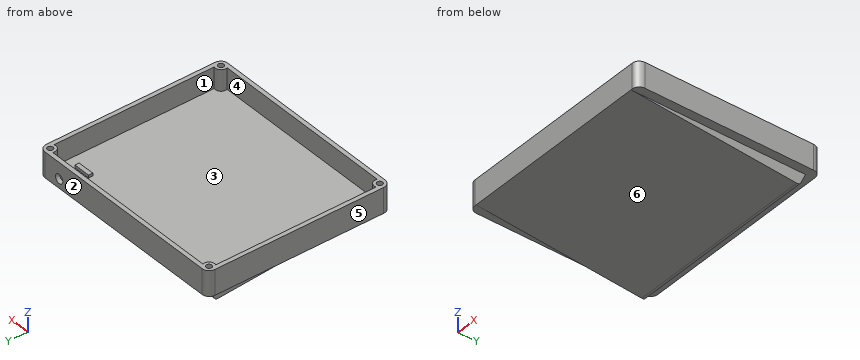
from build123d import *

# Parameters (mm, degrees)
LEFT_BODY_PAD_DEPTH            = 18
LEFT_BODY_CAVITY_POCKET_DEPTH  = 15
LEFT_BODY_BOSSES_R             = 4
LEFT_BODY_BOSS_PAD_DEPTH       = 15
LEFT_BODY_INSERT_HOLES_R       = 2
LEFT_BODY_INSERT_POCKETS_DEPTH = 7
LEFT_BODY_REST_PAD_DEPTH       = 68.531175
LEFT_BODY_REST_FILLET_R        = 3
LEFT_JACK_HOLE_R               = 3.25
LEFT_JACK_HOLE_POCKET_DEPTH    = 3.2
LEFT_JACK_STOP_W               = 12
LEFT_JACK_STOP_H               = 3
LEFT_JACK_STOP_PAD_DEPTH       = 2


with BuildPart() as part:
    # Left_Body_Outline → Left_Body_Pad (new body)
    with BuildSketch(Plane.XY.offset(-18)):
        with BuildLine():
            Line((-0.38035, -5.791), (138.682, -5.791))
            ThreePointArc((138.682, -5.791), (142.217534, -4.326534), (143.682, -0.791))
            Line((143.682, -0.791), (143.682, 119.971))
            ThreePointArc((143.682, 119.971), (142.217534, 123.506534), (138.682, 124.971))
            Line((138.682, 124.971), (-0.38035, 124.971))
            ThreePointArc((-0.38035, 124.971), (-3.915884, 123.506534), (-5.38035, 119.971))
            Line((-5.38035, 119.971), (-5.38035, -0.791))
            ThreePointArc((-5.38035, -0.791), (-3.915884, -4.326534), (-0.38035, -5.791))
        make_face()
    extrude(amount=LEFT_BODY_PAD_DEPTH)

    # Left_Body_Cavity → Left_Body_Cavity_Pocket (cut)
    with BuildSketch(Plane.XY):
        with BuildLine():
            Line((-0.38035, -2.791), (138.682, -2.791))
            ThreePointArc((138.682, -2.791), (140.096214, -2.205214), (140.682, -0.791))
            Line((140.682, -0.791), (140.682, 119.971))
            ThreePointArc((140.682, 119.971), (140.096214, 121.385214), (138.682, 121.971))
            Line((138.682, 121.971), (-0.38035, 121.971))
            ThreePointArc((-0.38035, 121.971), (-1.794564, 121.385214), (-2.38035, 119.971))
            Line((-2.38035, 119.971), (-2.38035, -0.791))
            ThreePointArc((-2.38035, -0.791), (-1.794564, -2.205214), (-0.38035, -2.791))
        make_face()
    extrude(amount=-LEFT_BODY_CAVITY_POCKET_DEPTH, mode=Mode.SUBTRACT)

    # Left_Body_Bosses → Left_Body_Boss_Pad (join)
    with BuildSketch(Plane.XY.offset(-15)):
        with Locations((-1.08035, -1.491)):
            Circle(LEFT_BODY_BOSSES_R)
        with Locations((139.382, -1.491)):
            Circle(LEFT_BODY_BOSSES_R)
        with Locations((-1.08035, 120.671)):
            Circle(LEFT_BODY_BOSSES_R)
        with Locations((139.382, 120.671)):
            Circle(LEFT_BODY_BOSSES_R)
    extrude(amount=LEFT_BODY_BOSS_PAD_DEPTH)

    # Left_Body_Insert_Holes → Left_Body_Insert_Pockets (cut)
    with BuildSketch(Plane.XY):
        with Locations((-1.08035, -1.491)):
            Circle(LEFT_BODY_INSERT_HOLES_R)
        with Locations((139.382, -1.491)):
            Circle(LEFT_BODY_INSERT_HOLES_R)
        with Locations((-1.08035, 120.671)):
            Circle(LEFT_BODY_INSERT_HOLES_R)
        with Locations((139.382, 120.671)):
            Circle(LEFT_BODY_INSERT_HOLES_R)
    extrude(amount=-LEFT_BODY_INSERT_POCKETS_DEPTH, mode=Mode.SUBTRACT)

    # Left_Body_Rest → Left_Body_Rest_Pad (join, symmetric)
    with BuildSketch(Plane.YZ.offset(69.150825)):
        Polygon((-5.791, -18), (118.971, -18), (114.852748, -27.112629), align=None)
    extrude(amount=LEFT_BODY_REST_PAD_DEPTH, both=True)

    # Left_Body_Rest_Fillet
    left_body_rest_fillet_edges = [part.edges().sort_by_distance(p)[0] for p in [
        (69.150825, 114.852748, -27.112629),
    ]]
    fillet(left_body_rest_fillet_edges, radius=LEFT_BODY_REST_FILLET_R)

    # Left_Jack_Hole → Left_Jack_Hole_Pocket (cut)
    with BuildSketch(Plane.XZ.offset(-124.971)):
        with Locations((126.182, -11.5)):
            Circle(LEFT_JACK_HOLE_R)
    extrude(amount=LEFT_JACK_HOLE_POCKET_DEPTH, mode=Mode.SUBTRACT)

    # Left_Jack_Stop → Left_Jack_Stop_Pad (join)
    with BuildSketch(Plane.XY.offset(-15)):
        with Locations((126.182, 107.271)):
            Rectangle(LEFT_JACK_STOP_W, LEFT_JACK_STOP_H)
    extrude(amount=LEFT_JACK_STOP_PAD_DEPTH)


solid = part.part
Read the model definition and answer for the solid it produces. Units are mm, in the model's axes. Face numbers are marked on the shaded views. A direction names the side the tool comes from. Give positions to 0.01 mm unless a question says otherwise; leave off trailing zeros. Loops run counter-clockwise (first coordinate to the right, second up) from the corner with the lowest first, then second, coordinate; pieces in that order, holes last. Notation, with made-up numbers: (-30, 30) - (-1, 30) arc R27 ccw to (-1, 51) - close; hole circle Ø6 at (6.25, -20). An arc over 180 degrees is marked (long way). Answer as CSV lines item,"result". Start each with the question number.
1) Determine the mould class of the marked faces 3, 4, 5 and 6 for opening direction X: released by +X, released by -X, zero draft, split by the parting line, or undercut.
2) Find section D-D (z = -21.5). Write down the section's boundary in (x, y), then the cut area to 3 significant figures.
3) Each of these flat-tipped pins is pushed along its axis until it touches: pin 1 Ø4.5 at (x, y) = (138.5, -1.5) entering from +Z; pin 2 Ø10 at (x, y) = (98, 21) entering from +Z; pin 3 Ø2 at (x, y) = (-1.5, -2) entering from +Z; pin 4 Ø5 at (x, z) = (126.182, -11.5) entering from +Y. Where does it stop, or does it pass through?
4) Which of the six approach directions +Z, -Z, +X, -X, +Y, -Y give full straight-line access (tool end or side, diameter ignored) to the marked faces 1 and 2?
5) Find section B-B (z = -5.25). Write down the section's boundary in (x, y).
6) Find section A-A (x = 114.5). Write down the section's boundary in (y, z), then the cut area to 3 significant figures.
7) Straight lines are drawn through the part: L1, parallel to X at y = 51, z = -4.25; L2, parallel to Y at x = 74.5, z = -4.75; L3, parallel to Y at x = 126.5, z = -14. For each, find the intervals that lie inside material, in ascending order. Write a range as from..to.
8) Find section C-C (y = 64.5). Write down the section's boundary in (x, z), then the cut area to 3 significant figures.
Findings below:
1,face 3,"undercut"
1,face 4,"undercut"
1,face 5,"released by -X"
1,face 6,"zero draft"
2,outline,"(0.62, 40.55) - (137.68, 40.55) - (137.68, 117.39) - (0.62, 117.39) - close"
2,area,"10,500 mm^2"
3,pin 1,"z = 0"
3,pin 2,"z = -15"
3,pin 3,"z = -7"
3,pin 4,"y = 108.77"
4,face 1,"+Z"
4,face 2,"+Z, -Z, +X, -X, +Y"
5,outline,"(-5.38, -0.79) arc R5 ccw to (-0.38, -5.79) - (138.68, -5.79) arc R5 ccw to (143.68, -0.79) - (143.68, 119.97) arc R5 ccw to (138.68, 124.97) - (-0.38, 124.97) arc R5 ccw to (-5.38, 119.97) - close; hole circle Ø4 at (-1.08, -1.49); hole circle Ø4 at (-1.08, 120.67); hole (-2.38, 2.29) arc R4 cw to (2.7, -2.79) - (135.6, -2.79) arc R4 cw to (140.68, 2.29) - (140.68, 116.89) arc R4 cw to (135.6, 121.97) - (2.7, 121.97) arc R4 cw to (-2.38, 116.89) - close; hole circle Ø4 at (139.38, -1.49); hole circle Ø4 at (139.38, 120.67)"
6,outline,"(-5.79, -18) - (112.76, -26.95) arc R3 ccw to (115.72, -25.2) - (118.97, -18) - (124.97, -18) - (124.97, 0) - (121.97, 0) - (121.97, -15) - (-2.79, -15) - (-2.79, 0) - (-5.79, 0) - close"
6,area,"1,050 mm^2"
7,L1,"-5.38..-2.38, 140.68..143.68"
7,L2,"-5.79..-2.79, 121.97..124.97"
7,L3,"-5.79..-2.79, 105.77..108.77"
8,outline,"(-5.38, -18) - (0.62, -18) - (0.62, -23.31) - (137.68, -23.31) - (137.68, -18) - (143.68, -18) - (143.68, 0) - (140.68, 0) - (140.68, -15) - (-2.38, -15) - (-2.38, 0) - (-5.38, 0) - close"
8,area,"1,260 mm^2"
